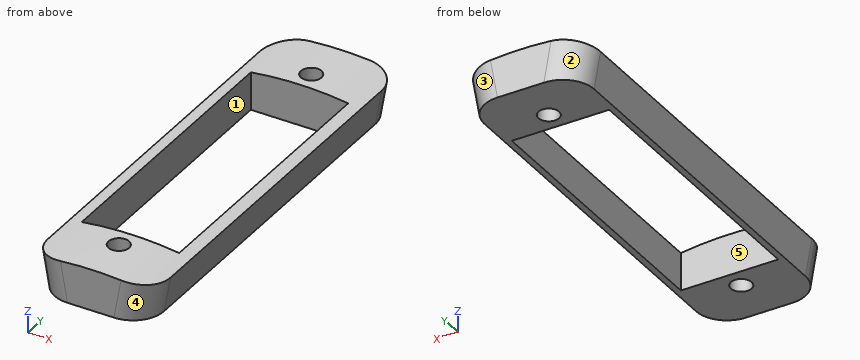
```python
from build123d import *

# Parameters (mm, degrees)
SKETCH1_W                         = 2
SKETCH1_H                         = 40
BULK_EXTRUDE_ANGLE                = 20
CONNECTOR_PASSTHRU_DEPTH          = 41.509013499
CONNECTOR_PASSTHRU_DEPTH_BACK     = 41.509013499
SKETCH2_R                         = 1
SKETCH2_W                         = 9.4
SKETCH2_H                         = 27.2
REAR_FLATTENING_REACH             = 42.509
SKETCH3_W                         = 11.10393272
SKETCH3_H                         = 40
SKETCH3_R                         = 1
SKETCH3_W_2                       = 9.4
SKETCH3_H_2                       = 27.2
REAR_FLATTENING_DIRECTION_2_DEPTH = 1.5
SKETCH4_W                         = 5.405389312
SKETCH4_H                         = 40
CUT_EXTRUDE2_DEPTH                = 42.783584431
SKETCH5_W                         = 5.359461023
SKETCH5_H                         = 40
CUT_EXTRUDE3_DEPTH                = 42.783584431
FILLET1_R                         = 3


with BuildPart() as part:
    # Sketch1 → BULK EXTRUDE (revolve, symmetric)
    with BuildSketch(Plane(origin=(0, 0, 0), x_dir=(0, 0, -1), z_dir=(1, 0, 0))) as bulk_extrude_sk:
        with Locations((1, 20)):
            Rectangle(SKETCH1_W, SKETCH1_H)
    revolve(axis=Axis((0, 0, -33.9725), (0, 1, 0)), revolution_arc=BULK_EXTRUDE_ANGLE / 2)
    revolve(bulk_extrude_sk.sketch, axis=Axis((0, 0, -33.9725), (0, -1, 0)), revolution_arc=BULK_EXTRUDE_ANGLE / 2)

    # Sketch2 → CONNECTOR PASSTHRU (cut, two sides: drawn at the far end of the back side and taken through both)
    with BuildSketch(Plane.XY.offset(-CONNECTOR_PASSTHRU_DEPTH_BACK)):
        with Locations((0, 4.52)):
            Circle(SKETCH2_R)
        with Locations((0, 35.48)):
            Circle(SKETCH2_R)
        with Locations((0, 20)):
            Rectangle(SKETCH2_W, SKETCH2_H)
    extrude(amount=CONNECTOR_PASSTHRU_DEPTH + CONNECTOR_PASSTHRU_DEPTH_BACK, mode=Mode.SUBTRACT)

    # Sketch3 → REAR FLATTENING (add, up to next)
    with BuildSketch(Plane.XY.offset(-2.485734117), mode=Mode.PRIVATE) as rear_flattening_sk1:
        with Locations((0, 20)):
            Rectangle(SKETCH3_W, SKETCH3_H)
        with Locations((0, 4.52)):
            Circle(SKETCH3_R, mode=Mode.SUBTRACT)
        with Locations((0, 35.48)):
            Circle(SKETCH3_R, mode=Mode.SUBTRACT)
        with Locations((0, 20)):
            Rectangle(SKETCH3_W_2, SKETCH3_H_2, mode=Mode.SUBTRACT)
    rear_flattening_tool1 = extrude(rear_flattening_sk1.sketch, amount=REAR_FLATTENING_REACH, mode=Mode.PRIVATE) - part.part
    add(rear_flattening_tool1.solids().sort_by_distance((0, 0.415126, -2.485734))[0])

    # Sketch3 → REAR FLATTENING direction 2 (add)
    with BuildSketch(Plane.XY.offset(-2.485734117)):
        with Locations((0, 20)):
            Rectangle(SKETCH3_W, SKETCH3_H)
        with Locations((0, 4.52)):
            Circle(SKETCH3_R, mode=Mode.SUBTRACT)
        with Locations((0, 35.48)):
            Circle(SKETCH3_R, mode=Mode.SUBTRACT)
        with Locations((0, 20)):
            Rectangle(SKETCH3_W_2, SKETCH3_H_2, mode=Mode.SUBTRACT)
    extrude(amount=-REAR_FLATTENING_DIRECTION_2_DEPTH)

    # Sketch4 → Cut-Extrude2 (cut, through all)
    with BuildSketch(Plane(origin=(5.80963966, 0, -1.02439622), x_dir=(-0.17364817766693075, 0, -0.9848077530122081), z_dir=(0.9848077530122081, 0, -0.17364817766693075))):
        with Locations((2.186576045, 20)):
            Rectangle(SKETCH4_W, SKETCH4_H)
    extrude(amount=CUT_EXTRUDE2_DEPTH, mode=Mode.SUBTRACT)

    # Sketch5 → Cut-Extrude3 (cut, through all)
    with BuildSketch(Plane(origin=(-5.80963966, 0, -1.02439622), x_dir=(-0.17364817766693072, 0, 0.9848077530122081), z_dir=(-0.9848077530122081, 0, -0.17364817766693072))):
        with Locations((-2.163611901, 20)):
            Rectangle(SKETCH5_W, SKETCH5_H)
    extrude(amount=CUT_EXTRUDE3_DEPTH, mode=Mode.SUBTRACT)

    # Fillet1
    fillet1_edges = [part.edges().sort_by_distance(p)[0] for p in [
        (5.593369303, 40, -2.250926364),
        (-5.593369303, 0, -2.250926364),
        (-5.593369303, 40, -2.250926364),
        (5.593369303, 0, -2.250926364),
    ]]
    fillet(fillet1_edges, radius=FILLET1_R)


solid = part.part
```
CAD build for the part. Positions are in the model's coordinates, mm. Face numbers are marked on the shaded views. A direction names the side the tool comes from. Give positions to 0.01 mm unless a question says otherwise; leave off trailing zeros. Order: outer loops, then holes, each group sorted by start corner. A loop starts at its lowest first (then second) coordinate and runs counter-clockwise, first axis right, second up.
(1) Saw through at B-B, the plane y = 17. Give the cut face in (x, z) (1 decimal), then the cut area to 3 significant figures.
(2) Saw through at A-A, the plane x = 0. Give the cut face in (y, z).
(3) Saw through at C-C, the plane y = 35.48. Give the cut face in (x, z) (1 decimal).
(4) Tool access for the marked faces 1 and 2: list every direction of +Z, -Z, +X, -X, +Y, -Y with a clear straight run to the whole face (end or side of a thin tool).
(5) Mould opens along Y. For the marked faces 3, 4 and 5 say: released by +Y, released by -Y, zero draft, split by the parting line, or undercut.
(6) Flat gauge pins, fed straight in: pin 1 (2 mm diameter, centred on x = 3.5, y = 8.5, fed in from -Z); pin 2 (2.5 mm diameter, centred on x = 0, y = 35.48, fed in from +Z); pin 3 (2 mm diameter, centred on y = 15, z = -2, fed in from +X); pin 4 (1.1 mm diameter, centred on y = 20.5, z = -1.5, fed in from -X). Where does each tip first touch, or does it go through?
(7) Drill centre lines: L1, parallel to Y at x = 0, z = -0.65; L2, parallel to Y at x = 0.5, z = -0.4; L3, parallel to Y at x = 1.5, z = -3.5. Where is each one in solid material? Low to high.
(8) Saw through at D-D, the plane z = -3.2. State how many separate pieces and enclosed holes the cut face has, then the cut area to 3 significant figures.
Results found:
1. outline: (-5.9, -0.5) - (-5.3, -4) - (-4.7, -4) - (-4.7, -0.3) arc R34 ccw to start; (4.7, -4) - (5.3, -4) - (5.9, -0.5) arc R34 ccw to (4.7, -0.3) - close
1. area: 6.44 mm2
2. outline: (0, -3.99) - (3.52, -3.99) - (3.52, 0) - (0, 0) - close; (5.52, -3.99) - (6.4, -3.99) - (6.4, 0) - (5.52, 0) - close; (33.6, -3.99) - (34.48, -3.99) - (34.48, 0) - (33.6, 0) - close; (36.48, -3.99) - (40, -3.99) - (40, 0) - (36.48, 0) - close
3. outline: (-5.9, -0.5) - (-5.3, -4) - (-1, -4) - (-1, 0) arc R34 ccw to start; (1, -4) - (5.3, -4) - (5.9, -0.5) arc R34 ccw to (1, 0) - close
4. face 1: +Z, -Z
4. face 2: -Z, -X, +Y
5. face 3: released by +Y
5. face 4: released by -Y
5. face 5: undercut
6. pin 1: passes through
6. pin 2: stops at z = 0
6. pin 3: stops at x = 5.81
6. pin 4: stops at x = -5.82
7. L1: y = 0 to 3.52, 5.52 to 6.4, 33.6 to 34.48, 36.48 to 40
7. L2: y = 0 to 3.65, 5.39 to 6.4, 33.6 to 34.61, 36.35 to 40
7. L3: y = 0 to 6.4, 33.6 to 40
8. separate pieces: 1
8. enclosed holes: 3
8. area: 164 mm2
